For this review, take the finished solid that the model builds, in its own axes (mm). Give positions to 0.01 mm unless a question says otherwise; leave off trailing zeros. Write each loop counter-clockwise with the first axis right and the second up, starting at its lowest first coordinate (ties: lowest second). Pieces come first, ordered by that corner, then holes. Notation, with made-up numbers: (26, 44) -> (63, 44) arc R22 cw to (63, 51) -> close; hole circle Ø5 at (-10, -35.5). An arc over 180 degrees is marked (long way). Write item = value, one per line.
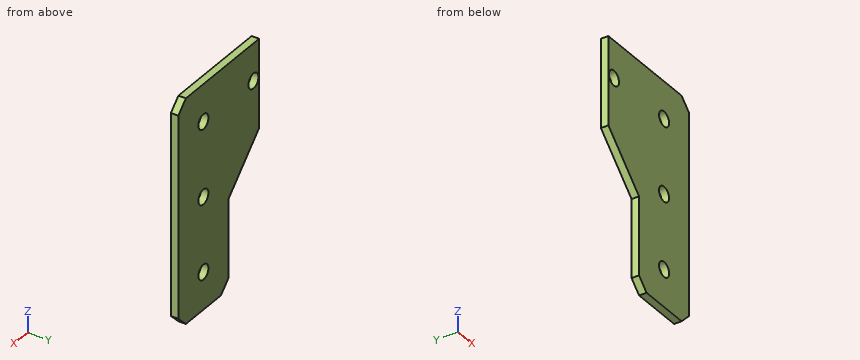
Autodesk Inventor part; units mm, degrees
ref_plane "YZ Plane" through (0, 0, 0) normal (1, 0, 0) x (0, 1, 0)
ref_plane "XZ Plane" through (0, 0, 0) normal (0, 1, 0) x (-1, 0, 0)
ref_plane "XY Plane" through (0, 0, 0) normal (0, 0, 1) x (1, 0, 0)
sketch "Sketch1" plane through (0, 0, 0) normal (0, 1, 0) x (-1, 0, 0)
  line L0 (25.4, -45.72) -> (45.72, -25.4)
  line L1 (0, -3.81) -> (3.81, 0)
  line L2 (3.81, -76.2) -> (0, -72.39)
  line L3 (21.59, -76.2) -> (25.4, -72.39)
  line L4 (0, -3.81) -> (0, -72.39)
  line L5 (3.81, -76.2) -> (21.59, -76.2)
  line L6 (25.4, -72.39) -> (25.4, -45.72)
  circle A0 centre (38.1, -12.7) radius 2.54
  circle A1 centre (12.7, -12.7) radius 2.54
  circle A2 centre (12.7, -38.1) radius 2.54
  circle A3 centre (12.7, -63.5) radius 2.54
  line L7 (45.72, -25.4) -> (45.72, 0)
  line L8 (45.72, 0) -> (3.81, 0)
  point P0 (0, 0)
extrude "Extrusion2" add sketch "Sketch1" along normal blind 2.54
sketch "Sketch2" plane through (-45.72, 0, -25.4) normal (-1, 0, 0) x (0, 0, 1)
  line L0 (31.6621, -8.1072) -> (-13.5147, -8.1072)
  line L1 (-13.5147, -8.1072) -> (-13.5147, 15.8231)
  line L2 (-13.5147, 15.8231) -> (31.6621, 15.8231)
  line L3 (31.6621, 15.8231) -> (31.6621, -8.1072)
  point P0 (25.4, 0)
extrude "Extrusion3" cut sketch "Sketch2" against normal blind 4.7625
properties part number "1in corner bracket for extrusions cut" material "Steel, Alloy"
(1) Take a section at C-C (z = -38.1). Write out the cut boundary in (x, y).
Answers below:
outline = (-33.02, 0) -> (-15.24, 0) -> (-15.24, 2.54) -> (-33.02, 2.54) -> close; (-10.16, 0) -> (0, 0) -> (0, 2.54) -> (-10.16, 2.54) -> close
(2) Take a section at B-B (x = -12.7). Write out the cut boundary in (y, z).
Answers below:
outline = (0, -76.2) -> (2.54, -76.2) -> (2.54, -66.04) -> (0, -66.04) -> close; (0, -60.96) -> (2.54, -60.96) -> (2.54, -40.64) -> (0, -40.64) -> close; (0, -35.56) -> (2.54, -35.56) -> (2.54, -15.24) -> (0, -15.24) -> close; (0, -10.16) -> (2.54, -10.16) -> (2.54, 0) -> (0, 0) -> close
(3) For pin 1 (1.5 mm diameter, centred on x = -24.5, y = 1, fed in from -Z); pin 2 (1.3 mm diameter, centred on y = 0.5, z = -61, fed in from -X), all flat-tipped, find the tip position at first contact; note any pin that passes through.
Answers below:
pin_1 = -74.04
pin_2 = -25.4
(4) Take a section at D-D (y = 1.85). Write out the cut boundary in (x, z), plus the area to 3 significant figures.
Answers below:
outline = (-40.96, -30.16) -> (-25.4, -45.72) -> (-25.4, -72.39) -> (-21.59, -76.2) -> (-3.81, -76.2) -> (0, -72.39) -> (0, -3.81) -> (-3.81, 0) -> (-40.96, 0) -> close; hole circle Ø5.08 at (-38.1, -12.7); hole circle Ø5.08 at (-12.7, -63.5); hole circle Ø5.08 at (-12.7, -38.1); hole circle Ø5.08 at (-12.7, -12.7)
area = 2,420 mm^2
(5) Take a section at A-A (x = -38.1). Write out the cut boundary in (y, z), plus the area to 3 significant figures.
Answers below:
outline = (0, -33.02) -> (2.54, -33.02) -> (2.54, -15.24) -> (0, -15.24) -> close; (0, -10.16) -> (2.54, -10.16) -> (2.54, 0) -> (0, 0) -> close
area = 71.0 mm^2
(6) To check wall thickness, follow probe 1 along Z at (x, y) = (-12.7, 1.4); probe 2 along Z at (x, y) = (-15, 2.4); probe 3 along X at (y, z) = (1.75, -51). State the ranges of each line that lie inside material, in increasing order.
Answers below:
probe_1 = -76.2 to -66.04, -60.96 to -40.64, -35.56 to -15.24, -10.16 to 0
probe_2 = -76.2 to -64.58, -62.42 to -39.18, -37.02 to -13.78, -11.62 to 0
probe_3 = -25.4 to 0
